```python
from build123d import *

# Parameters (mm, degrees)
BOSS_EXTRUDE1_DEPTH = 3.175
SKETCH2_W           = 1.5875
SKETCH2_H           = 3.175
CUT_EXTRUDE1_DEPTH  = 170.414546822
SKETCH3_R           = 3.175
CUT_EXTRUDE2_DEPTH  = 170.414546822
BOSS_EXTRUDE2_DEPTH = 9.525
SKETCH5_W           = 3.175
SKETCH5_H           = 80.645
CUT_EXTRUDE3_DEPTH  = 1.5875


with BuildPart() as part:
    # Sketch1 → Boss-Extrude1 (new body)
    with BuildSketch(Plane.XY):
        Polygon((89.265, 0), (148.955, 0), (148.955, 80.645), (0, 80.645), (0, 0), align=None)
    extrude(amount=BOSS_EXTRUDE1_DEPTH)

    # Sketch2 → Cut-Extrude1 (cut, through all)
    with BuildSketch(Plane(origin=(148.955, 0, 0), x_dir=(0, 0, -1), z_dir=(1, 0, 0))):
        with Locations((-2.38125, 20.6375)):
            Rectangle(SKETCH2_W, SKETCH2_H)
    extrude(amount=-CUT_EXTRUDE1_DEPTH, mode=Mode.SUBTRACT)

    # Sketch3 → Cut-Extrude2 (cut, through all)
    with BuildSketch(Plane.XY.offset(3.175)):
        with Locations((12.7, 34.925)):
            Circle(SKETCH3_R)
        with Locations((136.255, 34.925)):
            Circle(SKETCH3_R)
        with Locations((123.555, 34.925)):
            Circle(SKETCH3_R)
        with Locations((110.855, 34.925)):
            Circle(SKETCH3_R)
    extrude(amount=-CUT_EXTRUDE2_DEPTH, mode=Mode.SUBTRACT)

    # Sketch4 → Boss-Extrude2 (add)
    with BuildSketch(Plane(origin=(148.955, 0, 0), x_dir=(0, 0, -1), z_dir=(1, 0, 0))):
        Polygon((-3.175, 19.05), (-3.175, 0), (0, 0), (0, 80.645), (-3.175, 80.645), (-3.175, 22.225), (-1.5875, 22.225), (-1.5875, 19.05), align=None)
    extrude(amount=BOSS_EXTRUDE2_DEPTH)

    # Sketch5 → Cut-Extrude3 (cut)
    with BuildSketch(Plane.XY.offset(3.175)):
        with Locations((153.7175, 40.3225)):
            Rectangle(SKETCH5_W, SKETCH5_H)
    extrude(amount=-CUT_EXTRUDE3_DEPTH, mode=Mode.SUBTRACT)


solid = part.part
```
The listing builds one solid part. Answer for the finished solid, in the listing's coordinates (mm). Give positions to 0.01 mm unless a question says otherwise; leave off trailing zeros. Order: outer loops, then holes, each group sorted by start corner. A loop starts at its lowest first (then second) coordinate and runs counter-clockwise, first axis right, second up. Notation, with made-up numbers: M 34,-4 L 44,-4 A32 ccw 44,22 Z; hole C -34.5,-4.5 d5. An arc over 180 degrees is marked long. Put each result on its own line as item: value. Start each with the question number.
Item 1: For a pull along X with two mould halves and no side action, classify faces 1 (the face through (157, 10, 3.175)), 2 (the face through (0, 41, 2)), 3 (the face through (114, 20, 1.588)) as +X half, -X half, draft (parallel to the pull), parting line (faces both ways), or undercut.
Item 2: Find the intervals of material crossed by line 1 along Y through (x, z) = (12.7, 1.9) (3 decimals); line 2 along X through (y, z) = (16, 2.2) (3 decimals); line 3 along Y through (x, z) = (133.5, 2.15) (3 decimals), in increasing order.
Item 3: The part is cut by section B-B, the plane z = 2.4. Determine the outline of the cut face in (x, y) (3 decimals).
Answer key:
1. face 1: draft
1. face 2: -X half
1. face 3: undercut
2. line 1: y = 0 to 19.05, 22.225 to 31.75, 38.1 to 80.645
2. line 2: x = 0 to 152.13, 155.305 to 158.48
2. line 3: y = 0 to 19.05, 22.225 to 33.347, 36.503 to 80.645
3. outline: M 0,0 L 152.13,0 L 152.13,19.05 L 0,19.05 Z; M 0,22.225 L 152.13,22.225 L 152.13,80.645 L 0,80.645 Z; M 155.305,0 L 158.48,0 L 158.48,19.05 L 155.305,19.05 Z; M 155.305,22.225 L 158.48,22.225 L 158.48,80.645 L 155.305,80.645 Z; hole C 12.7,34.925 d6.35; hole C 110.855,34.925 d6.35; hole C 123.555,34.925 d6.35; hole C 136.255,34.925 d6.35
